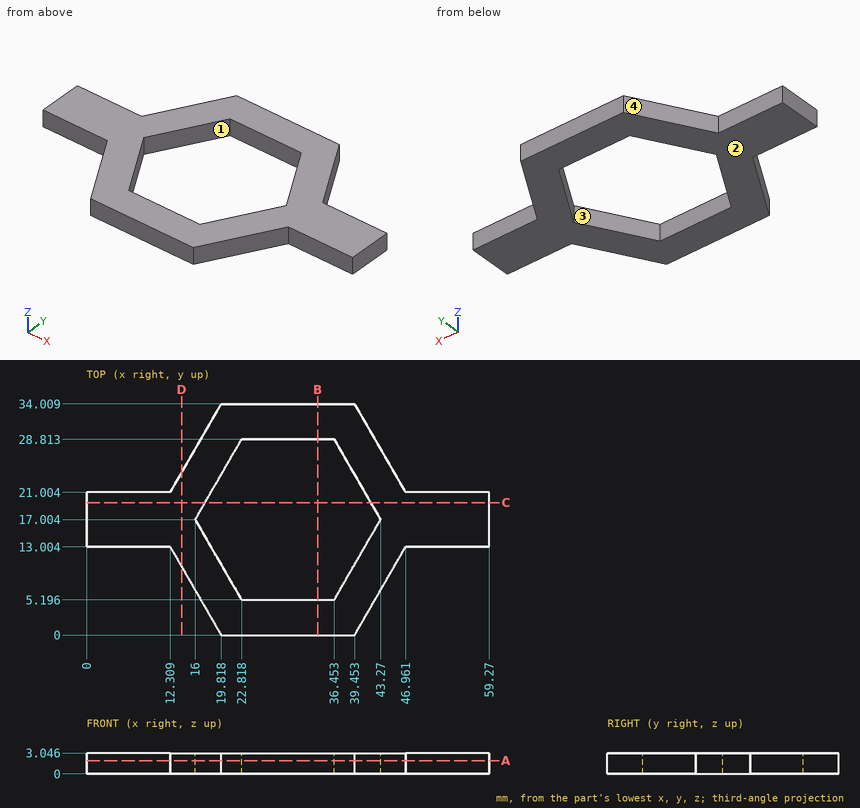
Could you check a few things on this drawing? It's one solid part, dimensions in mm from its lowest x, y, z. Give positions to 0.01 mm unless a question says otherwise; leave off trailing zeros. Write each loop counter-clockwise with the first axis right and the second up, starting at its lowest first coordinate (ties: lowest second). Pieces come first, ordered by that corner, then holes.
(1) Imagine slicing it at B-B, the plane x = 34. Write out the boundary of the cut face in (y, z).
Output values:
outline: (0, 0) - (5.2, 0) - (5.2, 3.05) - (0, 3.05) - close; (28.81, 0) - (34.01, 0) - (34.01, 3.05) - (28.81, 3.05) - close
(2) Imagine slicing it at D-D, the plane x = 14. Write out the boundary of the cut face in (y, z).
Output values:
outline: (10.08, 0) - (23.93, 0) - (23.93, 3.05) - (10.08, 3.05) - close
(3) Will these pins go through, and if not, where does the flat tip stop? pin 1 (1.5 mm diameter, centred on x = 50, z = 1.5, fed in from -Y); pin 2 (1.5 mm diameter, centred on x = 14, z = 1.5, fed in from -Y) (1 decimal); pin 3 (1.5 mm diameter, centred on x = 52, z = 1.5, fed in from +Y); pin 4 (6 mm diameter, centred on x = 22.5, y = 27, fed in from +Z).
Output values:
pin 1: stops at y = 13
pin 2: stops at y = 8.8
pin 3: stops at y = 21
pin 4: stops at z = 3.05
(4) If I drill on L1, parallel to Y at x = 31, z = 2.05; L2, parallel to Y at x = 37.5, z = 2.6 (1 decimal); L3, parallel to X at y = 11, z = 2.85 (1 decimal), over which ranges is the centre line in solid material (lowest first)?
Output values:
L1: y = 0 to 5.2, 28.81 to 34.01
L2: y = 0 to 7, 27 to 34
L3: x = 13.5 to 19.5, 39.8 to 45.8
(5) Imagine slicing it at A-A, the plane z = 1.95. Write out the boundary of the cut face in (x, y) (1 decimal), and give its area (3 significant figures).
Output values:
outline: (0, 13) - (12.3, 13) - (19.8, 0) - (39.5, 0) - (47, 13) - (59.3, 13) - (59.3, 21) - (47, 21) - (39.5, 34) - (19.8, 34) - (12.3, 21) - (0, 21) - close; hole (16, 17) - (22.8, 5.2) - (36.5, 5.2) - (43.3, 17) - (36.5, 28.8) - (22.8, 28.8) - close
area: 697 mm2
(6) Thinking about a two-plate mould opening in Y: for the marked faces 1, 2, 3 and 4, which applies, pulls with the +Y half, pulls with the -Y half, needs draft (parallel to the pull), parting line crosses it, or undercut?
Output values:
face 1: undercut
face 2: needs draft
face 3: undercut
face 4: pulls with the +Y half
(7) Imagine slicing it at C-C, the plane y = 19.5. Write out the boundary of the cut face in (x, z).
Output values:
outline: (0, 0) - (17.44, 0) - (17.44, 3.05) - (0, 3.05) - close; (41.83, 0) - (59.27, 0) - (59.27, 3.05) - (41.83, 3.05) - close
